For this review, use the dimensioned drawing (mm, ordinates from the lowest corner) and the shaded views. A direction names the side the tool comes from. Round coordinates to 2 decimals unless told otherwise and drop trailing zeros. Write each loop counter-clockwise with the first axis right and the second up, starting at its lowest first coordinate (ties: lowest second). Pieces come first, ordered by that corner, then holes.
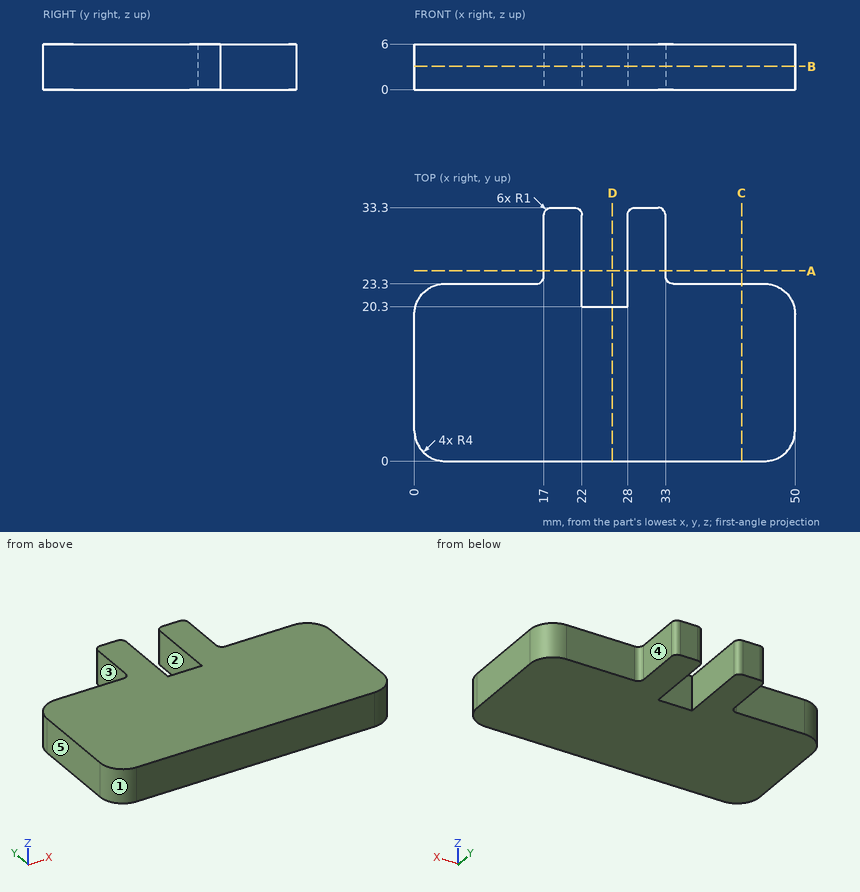
(1) We need section D-D, the plane x = 26. Give the boundary of the cut face in (y, z), and give its area (3 significant figures).
Geometry check:
outline: (0, 0) - (20.3, 0) - (20.3, 6) - (0, 6) - close
area: 122 mm2
(2) For line 1 along X through (y, z) = (29.5, 2.1); line 2 along Y through (x, z) = (15, 4.7); line 3 along X through (y, z) = (22, 4.45), list the stretches that pass through material, from the lowest coordinate up.
Geometry check:
line 1: x = 17 to 22, 28 to 33
line 2: y = 0 to 23.3
line 3: x = 1.05 to 22, 28 to 48.95
(3) For the marked faces 1, 2, 3, 4 and 5, list the 3-axis set-ups (+Z, -Z, +X, -X, +Y, -Y) from which the entire face can be reached by the end or side of a thin tool; tool diameter is ignored.
Geometry check:
face 1: +Z, -Z, -X, -Y
face 2: +Z, -Z, +Y
face 3: +Z, -Z, -X, +Y
face 4: +Z, -Z, +X, +Y
face 5: +Z, -Z, -X, +Y, -Y
(4) We need section B-B, the plane z = 3.05. Give the boundary of the cut face in (x, y), and give its area (3 significant figures).
Geometry check:
outline: (0, 4) arc R4 ccw to (4, 0) - (46, 0) arc R4 ccw to (50, 4) - (50, 19.3) arc R4 ccw to (46, 23.3) - (34, 23.3) arc R1 cw to (33, 24.3) - (33, 32.3) arc R1 ccw to (32, 33.3) - (29, 33.3) arc R1 ccw to (28, 32.3) - (28, 20.3) - (22, 20.3) - (22, 32.3) arc R1 ccw to (21, 33.3) - (18, 33.3) arc R1 ccw to (17, 32.3) - (17, 24.3) arc R1 cw to (16, 23.3) - (4, 23.3) arc R4 ccw to (0, 19.3) - close
area: 1,230 mm2
(5) We need section A-A, the plane y = 25. Give the boundary of the cut face in (x, z).
Geometry check:
outline: (17, 0) - (22, 0) - (22, 6) - (17, 6) - close; (28, 0) - (33, 0) - (33, 6) - (28, 6) - close
(6) For pin 1 Ø3 at (x, z) = (12.5, 3.5) entering from +Y; pin 2 Ø1.8 at (x, z) = (25, 4) entering from +Y; pin 3 Ø1.5 at (x, z) = (16, 1.5) entering from +Y, all flat-tipped, find the tip position at first contact; note any pin that passes through.
Geometry check:
pin 1: stops at y = 23.3
pin 2: stops at y = 20.3
pin 3: stops at y = 23.64
(7) We need section C-C, the plane x = 43. Give the boundary of the cut face in (y, z), and give its area (3 significant figures).
Geometry check:
outline: (0, 0) - (23.3, 0) - (23.3, 6) - (0, 6) - close
area: 140 mm2
